Input: dimensioned drawing with shaded views. Units: mm. Origin: part minimum x, y, z. Give positions to 0.01 mm unless a question says otherwise; leave off trailing zeros. Write each loop counter-clockwise with the first axis right and the second up, starting at its lowest first coordinate (ties: lowest second). Pieces come first, ordered by that corner, then holes. Notation, with made-up numbers: (56.5, 70.5) -> (68.5, 70.5) arc R26 ccw to (68.5, 102.5) -> close; hole circle Ø2 at (18.25, 87). An arc over 180 degrees is marked (long way). Return JSON: item names as keys, results as strings. Group by question number.
Item 1: Section B-B, the plane y = 7.5. Return loops of the section in (x, z) (1 decimal), then the cut area to 3 significant figures.
Item 2: Line query: line 1 (Z direction, x = 31.75, y = 5.25) (1 decimal); line 2 (Y direction, x = 18, z = 3) (1 decimal); line 3 (X direction, y = 11.25, z = 9.5) (1 decimal). Output: solid intervals per line, ascending. Write a range as [from, to].
Item 3: Section C-C, the plane x = 31.75. Return loops of the section in (y, z) (1 decimal).
Item 4: Mould query, pull axis X, two halves, no side actions, for the marked faces 1, 2 and 3. Classes: released by +X, released by -X, zero draft, split by the parting line, or undercut.
Item 5: Section A-A, the plane x = 44.5. Return loops of the section in (y, z) (1 decimal), then the cut area to 3 significant figures.
Item 6: Section D-D, the plane y = 2.5. Count the separate pieces of the cut face and the enclosed holes in it, then the cut area to 3 significant figures.
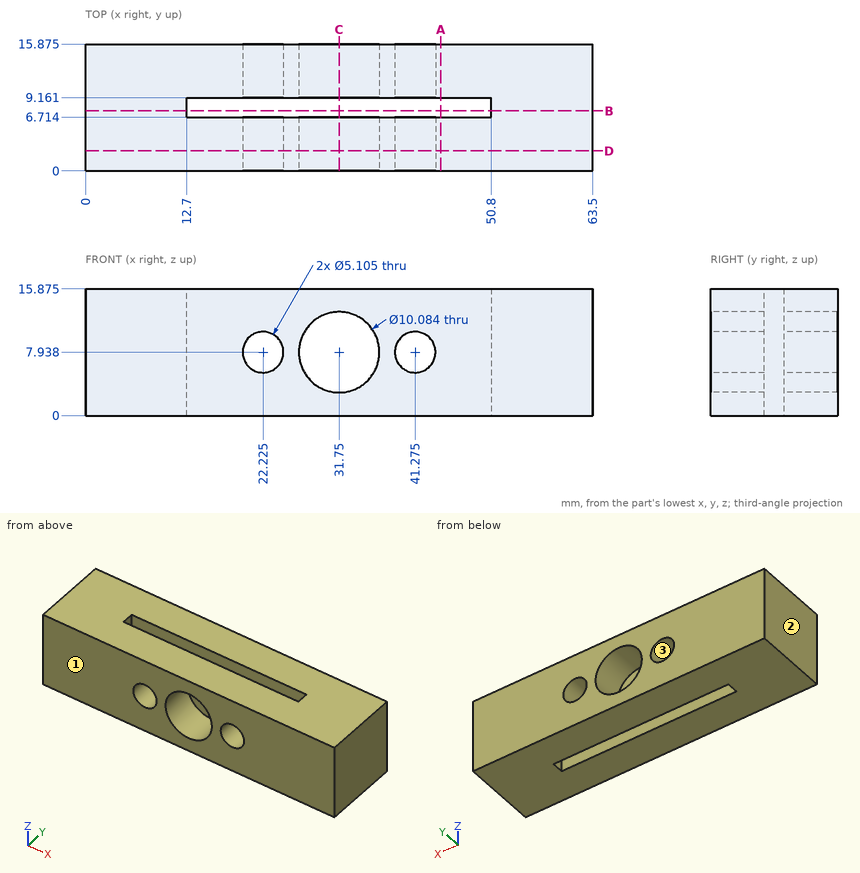
Answer below:
{
 "1": {"outline": "(0, 0) -> (12.7, 0) -> (12.7, 15.9) -> (0, 15.9) -> close; (50.8, 0) -> (63.5, 0) -> (63.5, 15.9) -> (50.8, 15.9) -> close", "area": "403 mm2"},
 "2": {"line 1": "z = [0, 2.9], [13, 15.9]", "line 2": "y = [0, 6.7], [9.2, 15.9]", "line 3": "x = [0, 20.2], [24.2, 27], [36.5, 39.3], [43.3, 63.5]"},
 "3": {"outline": "(0, 0) -> (6.7, 0) -> (6.7, 2.9) -> (0, 2.9) -> close; (0, 13) -> (6.7, 13) -> (6.7, 15.9) -> (0, 15.9) -> close; (9.2, 0) -> (15.9, 0) -> (15.9, 2.9) -> (9.2, 2.9) -> close; (9.2, 13) -> (15.9, 13) -> (15.9, 15.9) -> (9.2, 15.9) -> close"},
 "4": {"face 1": "zero draft", "face 2": "released by -X", "face 3": "undercut"},
 "5": {"outline": "(0, 0) -> (6.7, 0) -> (6.7, 15.9) -> (0, 15.9) -> close; (9.2, 0) -> (15.9, 0) -> (15.9, 15.9) -> (9.2, 15.9) -> close", "area": "213 mm2"},
 "6": {"separate pieces": "1", "enclosed holes": "3", "area": "887 mm2"}
}
